Work out the finished part from the listing and answer in its coordinate system (mm). Round coordinates to 2 decimals unless told otherwise and drop trailing zeros. Loops run counter-clockwise (first coordinate to the right, second up) from the corner with the lowest first, then second, coordinate; pieces in that order, holes last. Notation, with made-up numbers: (82.5, 31) - (87.5, 31) arc R15 ccw to (87.5, 47) - close; hole circle Ø1 at (-1.5, -31). An arc over 180 degrees is marked (long way). Answer as CSV lines item,"result". Start each with the question number.
Q1. Section D-D on y = 0 is taken. Write down the section's boundary in (x, z).
Q2. Section B-B on y = 40 is taken. Write down the section's boundary in (x, z), then the cut area to 3 significant figures.
Q3. Section C-C on z = 0.75 is taken. Write down the section's boundary in (x, y).
Q4. This flat-tipped pin is pushed along its axis until it touches: pin 1 Ø8 at (x, y) = (0, 32.5) entering from -Z. Where does it stop, or does it pass through?
Q5. Section A-A on x = 0 is taken. Write down the section's boundary in (y, z), then the cut area to 3 significant figures.
Q6. Straight lines are drawn through the part: L1, parallel to Y at x = 25, z = 0.75; L2, parallel to X at y = -3, z = 0.85; L3, parallel to X at y = -38.5, z = 1.2. For each, find the intervals that lie inside material, in ascending order. Write a range as [from, to].
```python
from build123d import *

# Parameters (mm, degrees)
F0_W     = 70
F0_H     = 100
F0_R     = 2
F1_DEPTH = 2


with BuildPart() as f1:
    # F0 (on Top) → F1 (new body)
    with BuildSketch(Plane.XY):
        Rectangle(F0_W, F0_H)
        with Locations((-25, -40)):
            Circle(F0_R, mode=Mode.SUBTRACT)
        with Locations((25, -40)):
            Circle(F0_R, mode=Mode.SUBTRACT)
        with Locations((-25, 0)):
            Circle(F0_R, mode=Mode.SUBTRACT)
        with Locations((-25, 40)):
            Circle(F0_R, mode=Mode.SUBTRACT)
        with BuildLine():
            ThreePointArc((-4.85, 0), (0, 4.85), (4.85, 0))
            ThreePointArc((4.85, 0), (0, -4.85), (-4.85, 0))
        make_face(mode=Mode.SUBTRACT)
        with Locations((25, 0)):
            Circle(F0_R, mode=Mode.SUBTRACT)
        with Locations((25, 40)):
            Circle(F0_R, mode=Mode.SUBTRACT)
    extrude(amount=F1_DEPTH)


solid = f1.part
```
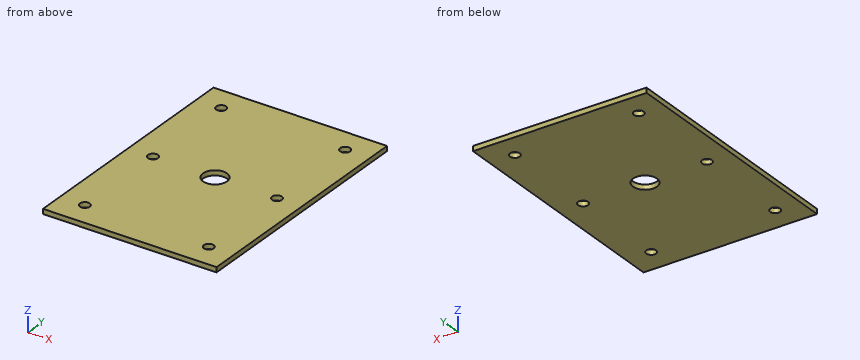
Findings:
1,outline,"(-35, 0) - (-27, 0) - (-27, 2) - (-35, 2) - close; (-23, 0) - (-4.85, 0) - (-4.85, 2) - (-23, 2) - close; (4.85, 0) - (23, 0) - (23, 2) - (4.85, 2) - close; (27, 0) - (35, 0) - (35, 2) - (27, 2) - close"
2,outline,"(-35, 0) - (-27, 0) - (-27, 2) - (-35, 2) - close; (-23, 0) - (23, 0) - (23, 2) - (-23, 2) - close; (27, 0) - (35, 0) - (35, 2) - (27, 2) - close"
2,area,"124 mm^2"
3,outline,"(-35, -50) - (35, -50) - (35, 50) - (-35, 50) - close; hole circle Ø4 at (-25, -40); hole circle Ø4 at (-25, 0); hole circle Ø4 at (-25, 40); hole circle Ø9.7 at (0, 0); hole circle Ø4 at (25, -40); hole circle Ø4 at (25, 0); hole circle Ø4 at (25, 40)"
4,pin 1,"stops at z = 0"
5,outline,"(-50, 0) - (-4.85, 0) - (-4.85, 2) - (-50, 2) - close; (4.85, 0) - (50, 0) - (50, 2) - (4.85, 2) - close"
5,area,"181 mm^2"
6,L1,"y = [-50, -42], [-38, -2], [2, 38], [42, 50]"
6,L2,"x = [-35, -3.81], [3.81, 35]"
6,L3,"x = [-35, -26.32], [-23.68, 23.68], [26.32, 35]"
